from build123d import *

# Parameters (mm, degrees)
SKETCH_1_W          = 100
SKETCH_1_H          = 80
EXTRUDE_1_DEPTH     = 10
SKETCH_2_R          = 3.3
CUT_EXTRUDE_1_DEPTH = 129.452325787
FILLET_1_R          = 5


with BuildPart() as part:
    # 草圖1 → 填料-伸長1 (new body)
    with BuildSketch(Plane(origin=(0, 0, 0), x_dir=(1, 0, 0), z_dir=(0, 1, 0))):
        with Locations((50, 40)):
            Rectangle(SKETCH_1_W, SKETCH_1_H)
    extrude(amount=EXTRUDE_1_DEPTH)

    # 草圖2 → 除料-伸長1 (cut, through all)
    with BuildSketch(Plane(origin=(0, 0, 0), x_dir=(1, 0, 0), z_dir=(0, 1, 0))):
        with Locations(Location((10, 10, 0), (0, 0, 270))):
            Circle(SKETCH_2_R)
        with Locations(Location((90, 10, 0), (0, 0, 270))):
            Circle(SKETCH_2_R)
        with Locations(Location((10, 70, 0), (0, 0, 270))):
            Circle(SKETCH_2_R)
        with Locations(Location((90, 70, 0), (0, 0, 270))):
            Circle(SKETCH_2_R)
    extrude(amount=CUT_EXTRUDE_1_DEPTH, mode=Mode.SUBTRACT)

    # 圓角1
    fillet_1_edges = [part.edges().sort_by_distance(p)[0] for p in [
        (0, 5, -80),
        (100, 5, -80),
        (100, 5, 0),
        (0, 5, 0),
    ]]
    fillet(fillet_1_edges, radius=FILLET_1_R)


solid = part.part
Geometry: final body of the model. Coordinates: model frame, mm. Give positions to 0.01 mm unless a question says otherwise; leave off trailing zeros. Write each loop counter-clockwise with the first axis right and the second up, starting at its lowest first coordinate (ties: lowest second). Pieces come first, ordered by that corner, then holes. Notation, with made-up numbers: (4.25, -23) -> (44.25, -23) arc R22 ccw to (44.25, -7) -> close; hole circle Ø5 at (52.25, 84.5). An arc over 180 degrees is marked (long way). Answer in a Markdown table with one row per item.
(1) Pin query (flat end, axial travel): pin 1 (5.5 mm diameter, centred on x = 90, z = -10, fed in from +Y). Return the tip coordinate at first contact, or that it passes through.
Answers below:
| item | result |
|---|---|
| pin 1 | through |
(2) Draft query along X for faces 1 (the flat face through (49, 0, -41)), 2 (the flat face through (0, 5, -40)), 3 (the cylindrical face through (10.1, 4.9, -73.3)). Return one class per face: +X half, -X half, draft (parallel to the pull), parting line (faces both ways), or undercut.
Answers below:
| item | result |
|---|---|
| face 1 | draft |
| face 2 | -X half |
| face 3 | undercut |
(3) Ray query, line 1 along Z through (x, y) = (90, 4); line 2 along X through (y, z) = (2, -70); line 3 along Z through (x, y) = (11, 9.5). Return the intervals inside material, ascending. Write a range as [from, to].
Answers below:
| item | result |
|---|---|
| line 1 | [-80, -73.3], [-66.7, -13.3], [-6.7, 0] |
| line 2 | [0, 6.7], [13.3, 86.7], [93.3, 100] |
| line 3 | [-80, -73.14], [-66.86, -13.14], [-6.86, 0] |
(4) Section query C-C on x = 10. Return loops of the section in (y, z).
Answers below:
| item | result |
|---|---|
| outline | (0, -80) -> (10, -80) -> (10, -73.3) -> (0, -73.3) -> close; (0, -66.7) -> (10, -66.7) -> (10, -13.3) -> (0, -13.3) -> close; (0, -6.7) -> (10, -6.7) -> (10, 0) -> (0, 0) -> close |
(5) Section query B-B on y = 5.25. Return loops of the section in (x, z).
Answers below:
| item | result |
|---|---|
| outline | (0, -75) arc R5 ccw to (5, -80) -> (95, -80) arc R5 ccw to (100, -75) -> (100, -5) arc R5 ccw to (95, 0) -> (5, 0) arc R5 ccw to (0, -5) -> close; hole circle Ø6.6 at (10, -70); hole circle Ø6.6 at (10, -10); hole circle Ø6.6 at (90, -70); hole circle Ø6.6 at (90, -10) |
(6) Section query A-A on z = -70. Return loops of the section in (x, y).
Answers below:
| item | result |
|---|---|
| outline | (0, 0) -> (6.7, 0) -> (6.7, 10) -> (0, 10) -> close; (13.3, 0) -> (86.7, 0) -> (86.7, 10) -> (13.3, 10) -> close; (93.3, 0) -> (100, 0) -> (100, 10) -> (93.3, 10) -> close |
